Geometry: final body of the model. Coordinates: model frame, mm. A direction names the side the tool comes from. Round coordinates to 2 decimals unless told otherwise and drop trailing zeros. Loops run counter-clockwise (first coordinate to the right, second up) from the corner with the lowest first, then second, coordinate; pieces in that order, holes last. Notation, with made-up numbers: M -22.75,68.25 L 0.25,68.25 A25 cw 0.25,91.25 Z; hole C 7.25,78.5 d9. An arc over 180 degrees is marked long. Return JSON: item names as keys, results as strings.
from build123d import *

# Parameters (mm, degrees)
SKETCH1_R           = 14.5
SKETCH1_R_2         = 9.5
BOSS_EXTRUDE1_DEPTH = 25
SKETCH2_R           = 1.5
BOSS_EXTRUDE2_DEPTH = 10
CIRPATTERN1_COUNT   = 6
SKETCH3_R           = 10.5
CUT_EXTRUDE1_DEPTH  = 5
CHAMFER1_SIZE       = 1
CHAMFER2_SIZE       = 1
SKETCH5_R           = 3
CUT_EXTRUDE2_DEPTH  = 32


with BuildPart() as part:
    # Sketch1 → Boss-Extrude1 (new body)
    with BuildSketch(Plane(origin=(0, 0, 0), x_dir=(1, 0, 0), z_dir=(0, 1, 0))):
        with Locations(Location((0, 0, 0), (0, 0, 270))):
            Circle(SKETCH1_R)
        with Locations(Location((0, 0, 0), (0, 0, 270))):
            Circle(SKETCH1_R_2, mode=Mode.SUBTRACT)
    extrude(amount=BOSS_EXTRUDE1_DEPTH)

    # Sketch2 → Boss-Extrude2 (add)
    with BuildSketch(Plane.XZ):
        with BuildLine():
            Line((-3, 13.002684968), (-3, 17.5))
            ThreePointArc((-3, 17.5), (0, 20.5), (3, 17.5))
            Line((3, 17.5), (3, 13.002684968))
            Line((3, 13.002684968), (-3, 13.002684968))
        make_face()
        with Locations(Location((0, 17.5, 0), (0, 0, 270))):
            Circle(SKETCH2_R, mode=Mode.SUBTRACT)
    boss_extrude2 = extrude(amount=-BOSS_EXTRUDE2_DEPTH)

    # CirPattern1: Boss-Extrude2 ×6 about axis
    cirpattern1_axis = Axis((0, 0, 0), (0, 1, 0))
    for i in range(1, CIRPATTERN1_COUNT):
        add(boss_extrude2.rotate(cirpattern1_axis, i * 360 / CIRPATTERN1_COUNT))

    # Sketch3 → Cut-Extrude1 (cut)
    with BuildSketch(Plane(origin=(0, 25, 0), x_dir=(1, 0, 0), z_dir=(0, 1, 0))):
        with Locations(Location((0, 0, 0), (0, 0, 270))):
            Circle(SKETCH3_R)
    extrude(amount=-CUT_EXTRUDE1_DEPTH, mode=Mode.SUBTRACT)

    # Chamfer1
    chamfer1_edges = [part.edges().sort_by_distance(p)[0] for p in [
        (0, 25, -10.5),
    ]]
    chamfer(chamfer1_edges, length=CHAMFER1_SIZE)

    # Chamfer2
    chamfer2_edges = [part.edges().sort_by_distance(p)[0] for p in [
        (0, 25, -14.5),
    ]]
    chamfer(chamfer2_edges, length=CHAMFER2_SIZE)

    # Sketch5 → Cut-Extrude2 (cut)
    with BuildSketch(Plane(origin=(7.25, 25, 12.557368355), x_dir=(0.8660254037844379, 0, -0.5000000000000013), z_dir=(0.5000000000000013, 0, 0.8660254037844379))):
        with Locations((0, -15)):
            Circle(SKETCH5_R)
    extrude(amount=-CUT_EXTRUDE2_DEPTH, mode=Mode.SUBTRACT)


solid = part.part
Q1. Section query B-B (x = 0). Output: boundary loops of the cut face in (y, z), plus the area to 3 significant figures.
Determined:
{"outline": "M 0,-20.5 L 10,-20.5 L 10,-19 L 0,-19 Z; M 0,-16 L 10,-16 L 10,-14.5 L 24,-14.5 L 25,-13.5 L 25,-11.5 L 24,-10.5 L 20,-10.5 L 20,-9.5 L 0,-9.5 Z; M 0,9.5 L 20,9.5 L 20,10.5 L 24,10.5 L 25,11.5 L 25,13.5 L 24,14.5 L 10,14.5 L 10,16 L 0,16 Z; M 0,19 L 10,19 L 10,20.5 L 0,20.5 Z", "area": "298 mm^2"}
Q2. Material intervals for L1, parallel to X at y = 2.75, z = -10; L2, parallel to X at y = 7, z = -17.5; L3, parallel to Z at x = 16.5, y = 6, sorted ascending.
Determined:
{"L1": "x = -17.88 to -15.98, -14.33 to -11.32, -10.5 to 10.5, 11.32 to 14.33, 15.98 to 17.88", "L2": "x = -3 to -1.5, 1.5 to 3", "L3": "z = -11.43 to -9.41, -8.09 to -6.06, 6.06 to 8.09, 9.41 to 11.43"}
Q3. Pull-direction query (Z, two-part tool) for faces 1 (the flat face through (-3, 5, -16)), 2 (the flat face through (-9, 20, -5)), 3 (the flat face through (12.24, 4.93, -10.53)); classes: pulls with the +Z half, pulls with the -Z half, needs draft (parallel to the pull), parting line crosses it, or undercut.
Determined:
{"face 1": "needs draft", "face 2": "undercut", "face 3": "pulls with the -Z half"}
Q4. Section query A-A (z = 0). Output: boundary loops of the cut face in (x, y).
Determined:
{"outline": "M -14.5,0 L -9.5,0 L -9.5,20 L -10.5,20 L -10.5,24 L -11.5,25 L -13.5,25 L -14.5,24 Z; M 9.5,0 L 14.5,0 L 14.5,24 L 13.5,25 L 11.5,25 L 10.5,24 L 10.5,20 L 9.5,20 Z"}
Q5. Pin query (flat end, axial travel): pin 1 (3.5 mm diameter, centred on x = 15, z = 6.5, fed in from +Y); pin 2 (12 mm diameter, centred on y = 18.5, z = 14.5, fed in from -X); pin 3 (1.5 mm diameter, centred on x = 7.5, y = 14, fed in from -Z). Return the tip coordinate at first contact, or that it passes through.
Determined:
{"pin 1": "stops at y = 10", "pin 2": "stops at x = -11.75", "pin 3": "stops at z = -12.83"}
Q6. Section query C-C (y = 12.5). Output: boundary loops of the cut face in (x, z).
Determined:
{"outline": "M -8.64,-11.65 L -6.11,-7.27 A9.5 cw 3.24,8.93 L 5.77,13.3 A14.5 ccw Z; M -5.77,-13.3 A14.5 ccw 8.64,11.65 L 6.11,7.27 A9.5 cw -3.24,-8.93 Z"}
Q7. Reachability of faces 4 (the flat face through (-12.2, 4.93, -10.51)), 5 (the flat face through (13.5, 10, 8.5)), 6 (the flat face through (12.2, 4.93, 10.51)), 7 (the flat face through (14, 10, -7)), 8 (the flat face through (-14, 10, 7)) from +Z, -Z, +X, -X, +Y, -Y: full face, straight path, thin tool, end or side. Return the list, or none.
Determined:
{"face 4": "-Z, +Y, -Y", "face 5": "+Z, +X, +Y", "face 6": "+Z, +Y, -Y", "face 7": "-Z, +X, +Y", "face 8": "+Z, -X, +Y"}
Q8. Section query D-D (y = 18). Output: boundary loops of the cut face in (x, z).
Determined:
{"outline": "C 0,0 d29; hole C 0,0 d19"}
